```python
from build123d import *

# Parameters (mm, degrees)
EXTRUDE_3_DEPTH     = 8.5
EXTRUDE_3_2_DEPTH   = 8.5
SKETCH_4_W          = 180.5019154
SKETCH_4_H          = 131.300307
EXTRUDE_5_DEPTH     = 10
EXTRUDE_6_DEPTH     = 5
SKETCH_8_W          = 25
SKETCH_8_H          = 6
CUT_EXTRUDE_1_DEPTH = 3.5
SKETCH_9_R          = 2.5
EXTRUDE_7_DEPTH     = 5
EXTRUDE_7_2_DEPTH   = 5
EXTRUDE_7_3_DEPTH   = 5
EXTRUDE_7_4_DEPTH   = 5
EXTRUDE_8_DEPTH     = 180.5019154


with BuildPart() as part:
    # Model → Extrude 3 (new body)
    with BuildSketch(Plane.XY):
        Polygon((565.397621393, -28.479593633), (562.397621393, -28.479593633), (562.397621393, -73.105300633), (393.895705993, -73.105300633), (393.895705993, -28.478893633), (390.895705993, -28.478893633), (390.895705993, -76.105300633), (565.397621393, -76.105300633), align=None)
    extrude(amount=EXTRUDE_3_DEPTH)



with BuildPart() as body_2:
    # Model → Extrude 3 2 (new body)
    with BuildSketch(Plane.XY):
        Polygon((393.895705993, -22.478893633), (393.895705993, 46.195006367), (562.397621393, 46.195006367), (562.397621393, -22.479593633), (565.397621393, -22.479593633), (565.397621393, 49.195006367), (390.895705993, 49.195006367), (390.895705993, -22.478893633), align=None)
    extrude(amount=EXTRUDE_3_2_DEPTH)


with BuildPart() as part_1:
    add(part.part)

    add(body_2.part)  # Extrude 5 merges body 2
    # Sketch 4 → Extrude 5 (add)
    with BuildSketch(Plane(origin=(0, 0, 0), x_dir=(-1, 0, 0), z_dir=(0, 0, -1))):
        with Locations((-478.146663693, -13.455147133)):
            Rectangle(SKETCH_4_W, SKETCH_4_H)
        with BuildLine():
            ThreePointArc((-562.397621393, -28.479593633), (-559.397621393, -25.479593633), (-562.397621393, -22.479593633))
            Line((-562.397621393, -22.479593633), (-565.397621393, -22.479593633))
            Line((-565.397621393, -22.479593633), (-565.397621393, 49.195006367))
            Line((-565.397621393, 49.195006367), (-390.895705993, 49.195006367))
            Line((-390.895705993, 49.195006367), (-390.895705993, -22.478893633))
            Line((-390.895705993, -22.478893633), (-393.895705993, -22.478893633))
            ThreePointArc((-393.895705993, -22.478893633), (-396.895705993, -25.478893633), (-393.895705993, -28.478893633))
            Line((-393.895705993, -28.478893633), (-390.895705993, -28.478893633))
            Line((-390.895705993, -28.478893633), (-390.895705993, -76.105300633))
            Line((-390.895705993, -76.105300633), (-565.397621393, -76.105300633))
            Line((-565.397621393, -76.105300633), (-565.397621393, -28.479593633))
            Line((-565.397621393, -28.479593633), (-562.397621393, -28.479593633))
        make_face(mode=Mode.SUBTRACT)
    extrude(amount=-EXTRUDE_5_DEPTH)

    # Sketch 5 → Extrude 6 (add)
    with BuildSketch(Plane(origin=(0, 0, 0), x_dir=(-1, 0, 0), z_dir=(0, 0, -1))):
        with BuildLine():
            Line((-562.397621393, 46.195006367), (-562.397621393, -22.479593633))
            ThreePointArc((-562.397621393, -22.479593633), (-561.327155124, -22.677076556), (-560.397621393, -23.243525656))
            Line((-560.397621393, -23.243525656), (-560.397621393, 44.195006367))
            Line((-560.397621393, 44.195006367), (-395.895705993, 44.195006367))
            Line((-395.895705993, 44.195006367), (-395.895705993, -23.242825656))
            ThreePointArc((-395.895705993, -23.242825656), (-394.966172262, -22.676376556), (-393.895705993, -22.478893633))
            Line((-393.895705993, -22.478893633), (-393.895705993, 46.195006367))
            Line((-393.895705993, 46.195006367), (-562.397621393, 46.195006367))
        make_face()
        with BuildLine():
            Line((-560.397621393, -71.105300633), (-560.397621393, -27.715661611))
            ThreePointArc((-560.397621393, -27.715661611), (-561.327155124, -28.28211071), (-562.397621393, -28.479593633))
            Line((-562.397621393, -28.479593633), (-562.397621393, -73.105300633))
            Line((-562.397621393, -73.105300633), (-393.895705993, -73.105300633))
            Line((-393.895705993, -73.105300633), (-393.895705993, -28.478893633))
            ThreePointArc((-393.895705993, -28.478893633), (-394.966172262, -28.28141071), (-395.895705993, -27.714961611))
            Line((-395.895705993, -27.714961611), (-395.895705993, -71.105300633))
            Line((-395.895705993, -71.105300633), (-560.397621393, -71.105300633))
        make_face()
    extrude(amount=-EXTRUDE_6_DEPTH)

    # Sketch 8 → Cut-Extrude 1 (cut)
    with BuildSketch(Plane.XY.offset(5)):
        with Locations((544.897621393, 49.195006367)):
            Rectangle(SKETCH_8_W, SKETCH_8_H)
    extrude(amount=CUT_EXTRUDE_1_DEPTH, mode=Mode.SUBTRACT)



with BuildPart() as body_2_2:
    # Sketch 9 → Extrude 7 (new body)
    with BuildSketch(Plane(origin=(0, 0, 0), x_dir=(-1, 0, 0), z_dir=(0, 0, -1))):
        with Locations((-430.805705993, -44.525300633)):
            Circle(SKETCH_9_R)
    extrude(amount=-EXTRUDE_7_DEPTH)


with BuildPart() as body_3:
    # Sketch 9 → Extrude 7 2 (new body)
    with BuildSketch(Plane(origin=(0, 0, 0), x_dir=(-1, 0, 0), z_dir=(0, 0, -1))):
        with Locations((-537.477621393, -44.525300633)):
            Circle(SKETCH_9_R)
    extrude(amount=-EXTRUDE_7_2_DEPTH)


with BuildPart() as body_4:
    # Sketch 9 → Extrude 7 3 (new body)
    with BuildSketch(Plane(origin=(0, 0, 0), x_dir=(-1, 0, 0), z_dir=(0, 0, -1))):
        with Locations((-421.895705993, 31.665006367)):
            Circle(SKETCH_9_R)
    extrude(amount=-EXTRUDE_7_3_DEPTH)


with BuildPart() as body_5:
    # Sketch 9 → Extrude 7 4 (new body)
    with BuildSketch(Plane(origin=(0, 0, 0), x_dir=(-1, 0, 0), z_dir=(0, 0, -1))):
        with Locations((-516.895705993, 31.665006367)):
            Circle(SKETCH_9_R)
    extrude(amount=-EXTRUDE_7_4_DEPTH)


with BuildPart() as part_2:
    add(part_1.part)

    add(body_2_2.part)  # Extrude 8 merges body 2 2

    add(body_3.part)  # Extrude 8 merges body 3

    add(body_4.part)  # Extrude 8 merges body 4

    add(body_5.part)  # Extrude 8 merges body 5
    # Sketch 10 → Extrude 8 (add)
    with BuildSketch(Plane.ZY.offset(-387.895705993)):
        Polygon((-1, -79.105300633), (-7.881157509, 52.195006367), (0, 52.195006367), (0, -79.105300633), align=None)
    extrude(amount=-EXTRUDE_8_DEPTH)


solid = part_2.part
```
Build history of the part. All positions in model axes, mm. A direction names the side the tool comes from. Coordinates: 2 decimals unless noted, no trailing zeros. Order: outer loops, then holes, each group sorted by start corner. A loop starts at its lowest first (then second) coordinate and runs counter-clockwise, first axis right, second up. Notation, with made-up numbers: (8.25, -1) -> (67.25, -1) arc R5 ccw to (67.25, 8) -> close; hole circle Ø8 at (65, -13). An arc over 180 degrees is marked (long way). Answer in a Markdown table with one row per item. Add a question column.
Q1. Band-saw the part on D-D, the plane y = -50.5. List the corners of the cut face in (x, z), then the cut area to 3 significant figures.
Q2. Which spindle directions (+Z, -Z, +X, -X, +Y, -Y) get a long thin tool onto all of the face, cutting with end or side? Do faces 1 (the face through (424.393, 31.775, 2.465)), 2 (the face through (532.398, 49, 7)). Say none if no direction does.
Q3. Mould opens along X. For faces 3 (the face through (538, -44, 5)), 4 (the face through (477, -79.105, 5)), 5 (the face through (387.896, -13, 3)) say: +X half, -X half, draft (parallel to the pull), parting line (faces both ways), or undercut.
Q4. Band-saw the part on A-A, the plane z = 2. List the corners of the cut face in (x, y) (3 decimals).
Q5. Band-saw the part on B-B, the plane x = 546.5. List the corners of the cut face in (y, z) (3 decimals), then the cut area to 3 significant figures.
Q6. Band-saw the part on C-C, the plane x = 470.5. List the corners of the cut face in (y, z) (3 decimals).
Q7. Drop flat-ended pins along their axis: pin 1 (4 mm diameter, centred on x = 422, y = 33, fed in from +Z); pin 2 (22.5 mm diameter, centred on x = 501, y = -53, fed in from +Z); pin 3 (1.5 mm diameter, centred on x = 550.5, y = 51, fed in from -Z). Give the stop position or say it passes through.
Q8. Wall check: line 1 along X through (y, z) = (-38.5, 4); line 2 along Y through (x, z) = (526.5, 8) (3 decimals); line 3 along Y through (x, z) = (539, 3.75) (3 decimals). Give the ranges that are in metal, low to high. Write a range as [from, to].
Answers follow:
| question | item | result |
|---|---|---|
| 1 | outline | (387.9, -2.5) -> (568.4, -2.5) -> (568.4, 10) -> (565.4, 10) -> (565.4, 8.5) -> (562.4, 8.5) -> (562.4, 5) -> (560.4, 5) -> (560.4, 0) -> (395.9, 0) -> (395.9, 5) -> (393.9, 5) -> (393.9, 8.5) -> (390.9, 8.5) -> (390.9, 10) -> (387.9, 10) -> close |
| 1 | area | 582 mm^2 |
| 2 | face 1 | +Z |
| 2 | face 2 | +Y |
| 3 | face 3 | undercut |
| 3 | face 4 | draft |
| 3 | face 5 | -X half |
| 4 | outline | (387.896, -79.105) -> (568.398, -79.105) -> (568.398, 52.195) -> (387.896, 52.195) -> close; circle Ø5 at (421.896, 31.665); circle Ø5 at (430.806, -44.525); circle Ø5 at (516.896, 31.665); circle Ø5 at (537.478, -44.525); hole (395.896, -71.105) -> (560.398, -71.105) -> (560.398, -27.716) arc R3 cw to (560.398, -23.244) -> (560.398, 44.195) -> (395.896, 44.195) -> (395.896, -23.243) arc R3 cw to (395.896, -27.715) -> close |
| 5 | outline | (-79.105, -1) -> (52.195, -7.881) -> (52.195, 5) -> (44.195, 5) -> (44.195, 0) -> (-71.105, 0) -> (-71.105, 5) -> (-73.105, 5) -> (-73.105, 8.5) -> (-76.105, 8.5) -> (-76.105, 10) -> (-79.105, 10) -> close; (49.195, 8.5) -> (52.195, 8.5) -> (52.195, 10) -> (49.195, 10) -> close |
| 5 | area | 693 mm^2 |
| 6 | outline | (-79.105, -1) -> (52.195, -7.881) -> (52.195, 10) -> (49.195, 10) -> (49.195, 8.5) -> (46.195, 8.5) -> (46.195, 5) -> (44.195, 5) -> (44.195, 0) -> (-71.105, 0) -> (-71.105, 5) -> (-73.105, 5) -> (-73.105, 8.5) -> (-76.105, 8.5) -> (-76.105, 10) -> (-79.105, 10) -> close |
| 7 | pin 1 | z = 5 |
| 7 | pin 2 | z = 0 |
| 7 | pin 3 | z = -7.86 |
| 8 | line 1 | [387.9, 395.9], [560.4, 568.4] |
| 8 | line 2 | [-79.105, -73.105], [46.195, 52.195] |
| 8 | line 3 | [-79.105, -71.105], [-46.508, -42.542], [44.195, 52.195] |
